from build123d import *

# Parameters (mm, degrees)
SKETCH_1_R               = 20
EXTRUDE_1_DEPTH          = 25
SKETCH_2_OUTSIDE_W       = 54.37
SKETCH_2_OUTSIDE_H       = 54.37
SKETCH_2_OUTSIDE_R       = 17.5
CUT_EXTRUDE_1_DEPTH      = 20
SKETCH_3_R               = 15.1
CUT_EXTRUDE_2_DEPTH      = 6
SKETCH_4_R               = 4
CUT_EXTRUDE_3_DEPTH      = 38.749172176
SKETCH_4_3_R             = 1.6
CUT_EXTRUDE_4_DEPTH      = 38.749172176
CUT_EXTRUDE_START        = 15
SKETCH_4_4_R             = 1.6
CUT_EXTRUDE_5_DEPTH      = 23.749172176
PATTERN_CIRCULAR_1_COUNT = 3
CHAMFER_1_SIZE           = 0.5
CHAMFER_2_SIZE           = 1
FILLET_1_R               = 0.6


with BuildPart() as part:
    # Sketch 1 → Extrude 1 (new body)
    with BuildSketch(Plane(origin=(0, 0, 0), x_dir=(1, 0, 0), z_dir=(0, 1, 0))):
        with Locations(Location((0, 0, 0), (0, 0, 270))):
            Circle(SKETCH_1_R)
    extrude(amount=EXTRUDE_1_DEPTH)

    # Sketch 2 outside → Cut-Extrude 1 (cut)
    with BuildSketch(Plane(origin=(0, 0, 0), x_dir=(1, 0, 0), z_dir=(0, 1, 0))):
        Rectangle(SKETCH_2_OUTSIDE_W, SKETCH_2_OUTSIDE_H)
        with Locations(Location((0, 0, 0), (0, 0, 270))):
            Circle(SKETCH_2_OUTSIDE_R, mode=Mode.SUBTRACT)
    extrude(amount=CUT_EXTRUDE_1_DEPTH, mode=Mode.SUBTRACT)

    # Sketch 3 → Cut-Extrude 2 (cut)
    with BuildSketch(Plane.XZ):
        with Locations(Location((0, 0, 0), (0, 0, 270))):
            Circle(SKETCH_3_R)
    extrude(amount=-CUT_EXTRUDE_2_DEPTH, mode=Mode.SUBTRACT)

    # Sketch 4 → Cut-Extrude 3 (cut, through all)
    with BuildSketch(Plane(origin=(0, 0, 0), x_dir=(1, 0, 0), z_dir=(0, 1, 0))):
        with Locations(Location((0, 0, 0), (0, 0, 90))):
            Circle(SKETCH_4_R)
    extrude(amount=CUT_EXTRUDE_3_DEPTH, mode=Mode.SUBTRACT)

    # Sketch 4_3 → Cut-Extrude 4 (cut, through all)
    with BuildSketch(Plane(origin=(0, 0, 0), x_dir=(1, 0, 0), z_dir=(0, 1, 0))):
        with Locations(Location((0, 12, 0), (0, 0, 90))):
            Circle(SKETCH_4_3_R)
    cut_extrude_4 = extrude(amount=CUT_EXTRUDE_4_DEPTH, mode=Mode.SUBTRACT)

    # Sketch 4_4 → Cut-Extrude 5 (cut, through all)
    with BuildSketch(Plane(origin=(0, 0, 0), x_dir=(1, 0, 0), z_dir=(0, 1, 0)).offset(CUT_EXTRUDE_START)):
        Polygon((2.85, 10.354551733), (2.85, 13.645448267), (0, 15.290896534), (-2.85, 13.645448267), (-2.85, 10.354551733), (0, 8.709103466), align=None)
        with Locations(Location((0, 12, 0), (0, 0, 90))):
            Circle(SKETCH_4_4_R, mode=Mode.SUBTRACT)
    cut_extrude_5 = extrude(amount=CUT_EXTRUDE_5_DEPTH, mode=Mode.SUBTRACT)

    # Pattern Circular 1: Cut-Extrude 4, Cut-Extrude 5 ×3 about axis
    pattern_circular_1_axis = Axis((0, 0, 0), (0, 1, 0))
    add([cut_extrude_4.rotate(pattern_circular_1_axis, i * 360 / PATTERN_CIRCULAR_1_COUNT) for i in range(1, PATTERN_CIRCULAR_1_COUNT)], mode=Mode.SUBTRACT)
    add([cut_extrude_5.rotate(pattern_circular_1_axis, i * 360 / PATTERN_CIRCULAR_1_COUNT) for i in range(1, PATTERN_CIRCULAR_1_COUNT)], mode=Mode.SUBTRACT)

    # Chamfer 1
    chamfer_1_edges = [part.edges().sort_by_distance(p)[0] for p in [
        (0, 25, -20),
        (0, 20, -20),
        (0, 0, -17.5),
    ]]
    chamfer(chamfer_1_edges, length=CHAMFER_1_SIZE)

    # Chamfer 2
    chamfer_2_edges = [part.edges().sort_by_distance(p)[0] for p in [
        (0, 6, 4),
        (0, 25, 4),
    ]]
    chamfer(chamfer_2_edges, length=CHAMFER_2_SIZE)

    # Fillet 1
    fillet_1_edges = [part.edges().sort_by_distance(p)[0] for p in [
        (0, 6, 15.1),
    ]]
    fillet(fillet_1_edges, radius=FILLET_1_R)


solid = part.part
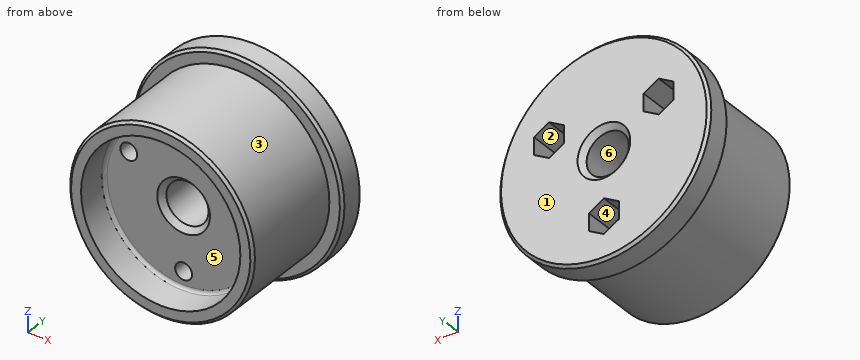
Geometry: final body of the model. Coordinates: model frame, mm. Face numbers are marked on the shaded views. A direction names the side the tool comes from. Round coordinates to 2 decimals unless told otherwise and drop trailing zeros. Loops run counter-clockwise (first coordinate to the right, second up) from the corner with the lowest first, then second, coordinate; pieces in that order, holes last. Notation, with made-up numbers: M 89,67.5 L 141,67.5 A32 cw 141,99.5 Z; hole C 23,49 d9. An arc over 180 degrees is marked long. Put each result on its own line as item: value. Start each with the question number.
(1) Contact query for flat-ended pins moving along their axis: pin 1 Ø1.6 at (y, z) = (18, 5.5) entering from +X; pin 2 Ø3.5 at (x, z) = (10.39, 6) entering from +Y; pin 3 Ø2.5 at (y, z) = (18, -12.5) entering from -X. Output: stop coordinate, or through.
(2) Section query B-B (y = 2). Return loops of the section in (x, z), then the cut area to 3 significant figures.
(3) Material intervals for line 1 along X through (y, z) = (11, 6); line 2 along X through (y, z) = (2.85, 0); line 3 along Y through (x, z) = (4.5, -3.5), sorted ascending. Write a range as [from, to].
(4) Draft query along X for the marked faces 1, 2 and 3. Return one class per face: +X half, -X half, draft (parallel to the pull), parting line (faces both ways), or undercut.
(5) Section query D-D (y = 6.5). Return loops of the section in (x, z), then the cut area to 3 significant figures.
(6) Set-up query: the marked faces 4, 5 and 6. Return all of +Z, -Z, +X, -X, +Y, -Y with unobstructed straight access to the full face (end or side cutting, diameter ignored); none if empty.
(7) Section query A-A (y = 9). Return loops of the section in (x, z), then the cut area to 3 significant figures.
(8) Section query C-C (z = 6). State how many separate pieces and enclosed holes the cut face has, then the cut area to 3 significant figures.
Findings below:
1. pin 1: stops at x = 16.86
1. pin 2: stops at y = 15
1. pin 3: stops at x = -13.4
2. outline: C 0,0 d35; hole C 0,0 d30.2
2. area: 246 mm2
3. line 1: x = [-16.44, -11.99], [-8.79, 8.79], [11.99, 16.44]
3. line 2: x = [-17.5, -15.1], [15.1, 17.5]
3. line 3: y = [6, 25]
4. face 1: draft
4. face 2: undercut
4. face 3: parting line
5. outline: C 0,0 d35; hole C -10.39,6 d3.2; hole C 0,0 d9; hole C 0,-12 d3.2; hole C 10.39,6 d3.2
5. area: 874 mm2
6. face 4: +Y
6. face 5: -Y
6. face 6: +Y, -Y
7. outline: C 0,0 d35; hole C -10.39,6 d3.2; hole C 0,0 d8; hole C 0,-12 d3.2; hole C 10.39,6 d3.2
7. area: 888 mm2
8. separate pieces: 3
8. enclosed holes: 0
8. area: 510 mm2
